Autodesk Inventor part; units mm, degrees
ref_plane "YZ Plane" through (0, 0, 0) normal (1, 0, 0) x (0, 1, 0)
ref_plane "XZ Plane" through (0, 0, 0) normal (0, 1, 0) x (-1, 0, 0)
ref_plane "XY Plane" through (0, 0, 0) normal (0, 0, 1) x (1, 0, 0)
sketch "スケッチ1" plane through (0, 0, 0) normal (0, 0, 1) x (1, 0, 0)
  circle A0 centre (0, 0) radius 6.25
  dimension "d0" = 12.5
extrude "押し出し1" add sketch "スケッチ1" along normal blind 115
sketch "スケッチ2" plane through (0, 0, 115) normal (0, 0, 1) x (1, 0, 0)
  line L0 (10, -10) -> (-10, -10)
  line L1 (-10, -10) -> (-10, 10)
  line L2 (-10, 10) -> (10, 10)
  line L3 (10, 10) -> (10, -10)
  line L4 (10, -10) -> (-10, 10) construction
  line L5 (-10, -10) -> (10, 10) construction
  point P0 (0, 0)
  dimension "d3" = 20
  dimension "d4" = 20
extrude "押し出し2" add sketch "スケッチ2" along normal blind 50
sketch "スケッチ3" plane through (0, 0, 165) normal (0, 0, 1) x (1, 0, 0)
  circle A0 centre (0, 0) radius 6.25
  dimension "d7" = 12.5
extrude "押し出し3" add sketch "スケッチ3" along normal blind 29
sketch "スケッチ4" plane through (0, 0, 194) normal (0, 0, 1) x (1, 0, 0)
  circle A0 centre (0, 0) radius 6.2
  dimension "d11" = 12.4
extrude "押し出し4" add sketch "スケッチ4" along normal blind 15 draft 2
sketch "スケッチ5" plane through (0, 0, 209) normal (0, 0, 1) x (1, 0, 0)
  circle A0 centre (0, 0) radius 6.7238
extrude "押し出し5" add sketch "スケッチ5" along normal blind 33 draft -10
properties part number "Coordinate"
Geometry: final body of the model. Coordinates: model frame, mm. A direction names the side the tool comes from. Give positions to 0.01 mm unless a question says otherwise; leave off trailing zeros. Write each loop counter-clockwise with the first axis right and the second up, starting at its lowest first coordinate (ties: lowest second). Pieces come first, ordered by that corner, then holes. Notation, with made-up numbers: M -1,73.5 L 49,73.5 A32 cw 49,101.5 Z; hole C 8.25,-39.5 d1. An arc over 180 degrees is marked long. Answer in a Markdown table with one row per item. Add a question column.
(1) Section B-B on z = 223. Return loops of the section in (x, y).
(2) Reachability of faces 1 (the cylindrical face through (5.96, -1.88, 56.7)), 2 (the flat face through (0, 0, 0)) from +Z, -Z, +X, -X, +Y, -Y: full face, straight path, thin tool, end or side. Return the list, or none.
(3) First-contact query: pin 1 (4 mm diameter, centred on y = 0.5, z = 30, fed in from +X); pin 2 (12 mm diameter, centred on y = 6.5, z = 204.5, fed in from +X); pin 3 (1 mm diameter, centred on y = 4.5, z = 84, fed in from -X); pin 4 (3 mm diameter, centred on x = 2.5, y = 4, fed in from -Z). Flat tips, straight axial feed; report the tip coordinate or a pass-through.
(4) Section A-A on z = 68. Return loops of the section in (x, y), and give its area (3 significant figures).
(5) Ray query, line 1 (Z direction, x = 2.25, y = 6.5); line 2 (X direction, y = -0.75, z = 192.5); line 3 (X direction, y = -2, z = 191). Return the intervals inside material, ascending.
(6) Mould query, pull axis Z, two halves, no side actions, for faces 3 (the flat face through (-10, 0, 140)), 4 (the cylindrical face through (5.96, -1.88, 179.3)), 5 (the flat face through (-5, 5, 115)), 6 (the conical face through (6.167, 1.942, 201.605)). Classes: +Z half, -Z half, draft (parallel to the pull), parting line (faces both ways), or undercut.
Result set:
| question | item | result |
|---|---|---|
| 1 | outline | C 0,0 d8.51 |
| 2 | face 1 | -Z |
| 2 | face 2 | -Z, +X, -X, +Y, -Y |
| 3 | pin 1 | stops at x = 6.25 |
| 3 | pin 2 | stops at x = 6.58 |
| 3 | pin 3 | stops at x = -4.8 |
| 3 | pin 4 | stops at z = 0 |
| 4 | outline | C 0,0 d12.5 |
| 4 | area | 123 mm^2 |
| 5 | line 1 | z = 115 to 165 |
| 5 | line 2 | x = -6.2 to 6.2 |
| 5 | line 3 | x = -5.92 to 5.92 |
| 6 | face 3 | draft |
| 6 | face 4 | undercut |
| 6 | face 5 | -Z half |
| 6 | face 6 | undercut |
